from build123d import *

# Parameters (mm, degrees)
SKETCH1_R           = 6.5
BOSS_EXTRUDE1_DEPTH = 22
CAVITY1_START       = 2
CAVITY1_OUTLINE_R   = 5
CAVITY1_OUTLINE_R_2 = 0.75
CAVITY1_DEPTH       = 20
CAVITY1_START_2     = 17
CAVITY1_2_OUTLINE_R = 0.75
CAVITY1_2_DEPTH     = 5
SKETCH2_R           = 0.3
CUT_EXTRUDE1_DEPTH  = 23.011360703


# Read off the part's stored shape, not the designer's step: Cavity1
with BuildPart() as part:
    # Sketch1 → Boss-Extrude1 (new body)
    with BuildSketch(Plane(origin=(0, 0, 0), x_dir=(1, 0, 0), z_dir=(0, 1, 0))):
        with Locations(Location((0, 0, 0), (0, 0, 270))):
            Circle(SKETCH1_R)
    extrude(amount=BOSS_EXTRUDE1_DEPTH)

    # Cavity1 outline → Cavity1 (cut)
    with BuildSketch(Plane(origin=(0, 0, 0), x_dir=(1, 0, 0), z_dir=(0, 1, 0)).offset(CAVITY1_START)):
        Circle(CAVITY1_OUTLINE_R)
        with BuildLine():
            ThreePointArc((-1.5, -2.598076211), (0, -3), (1.5, -2.598076211))
            Line((1.5, -2.598076211), (2, -3.464101615))
            ThreePointArc((2, -3.464101615), (0, -4), (-2, -3.464101615))
            Line((-2, -3.464101615), (-1.5, -2.598076211))
        make_face(mode=Mode.SUBTRACT)
        with BuildLine():
            ThreePointArc((-2.598076211, 1.5), (-3, 0), (-2.598076211, -1.5))
            Line((-2.598076211, -1.5), (-3.464101615, -2))
            ThreePointArc((-3.464101615, -2), (-4, 0), (-3.464101615, 2))
            Line((-3.464101615, 2), (-2.598076211, 1.5))
        make_face(mode=Mode.SUBTRACT)
        Circle(CAVITY1_OUTLINE_R_2, mode=Mode.SUBTRACT)
        with BuildLine():
            ThreePointArc((2.598076211, -1.5), (3, 0), (2.598076211, 1.5))
            Line((2.598076211, 1.5), (3.464101615, 2))
            ThreePointArc((3.464101615, 2), (4, 0), (3.464101615, -2))
            Line((3.464101615, -2), (2.598076211, -1.5))
        make_face(mode=Mode.SUBTRACT)
        with BuildLine():
            ThreePointArc((1.5, 2.598076211), (0, 3), (-1.5, 2.598076211))
            Line((-1.5, 2.598076211), (-2, 3.464101615))
            ThreePointArc((-2, 3.464101615), (0, 4), (2, 3.464101615))
            Line((2, 3.464101615), (1.5, 2.598076211))
        make_face(mode=Mode.SUBTRACT)
    extrude(amount=CAVITY1_DEPTH, mode=Mode.SUBTRACT)

    # Cavity1 2 outline → Cavity1 2 (cut)
    with BuildSketch(Plane(origin=(0, 0, 0), x_dir=(1, 0, 0), z_dir=(0, 1, 0)).offset(CAVITY1_START_2)):
        Circle(CAVITY1_2_OUTLINE_R)
    extrude(amount=CAVITY1_2_DEPTH, mode=Mode.SUBTRACT)

    # Sketch2 → Cut-Extrude1 (cut, through all)
    with BuildSketch(Plane(origin=(0, 2, 0), x_dir=(1, 0, 0), z_dir=(0, 1, 0))):
        with Locations(Location((0, 4.5, 0), (0, 0, 270))):
            Circle(SKETCH2_R)
        with Locations(Location((4.5, 0, 0), (0, 0, 270))):
            Circle(SKETCH2_R)
        with Locations(Location((0, -4.5, 0), (0, 0, 270))):
            Circle(SKETCH2_R)
        with Locations(Location((-4.5, 0, 0), (0, 0, 270))):
            Circle(SKETCH2_R)
    extrude(amount=-CUT_EXTRUDE1_DEPTH, mode=Mode.SUBTRACT)


solid = part.part
The listing builds one solid part. Answer for the finished solid, in the listing's coordinates (mm). A direction names the side the tool comes from. Coordinates: 2 decimals unless noted, no trailing zeros. Loops run counter-clockwise (first coordinate to the right, second up) from the corner with the lowest first, then second, coordinate; pieces in that order, holes last.
1) Determine the mould class of faces 3 (the face through (-3.955, 10.846, -5.158)), 4 (the face through (-3, 12, 0)), 5 (the face through (-3.4, 22, 0)) for opening direction X: pulls with the +X half, pulls with the -X half, needs draft (parallel to the pull), parting line crosses it, or undercut.
2) Find section B-B on z = 0. Write down the section's boundary in (x, y).
3) Find section A-A on y = 14.5. Write down the section's boundary in (x, z).
4) Find the intervals of material crossed by L1, parallel to X at y = 14, z = 0; L2, parallel to X at y = 0.75, z = 0; L3, parallel to Z at x = 1, y = 3, in increasing order.
5) Find section D-D on x = -4.5. Write down the section's boundary in (y, z), then the cut area to 3 significant figures.
6) A tool of negligible diameter and unlimited length cuts with its end or side. For faces 1 (the face through (1.754, 11.86, -3.037)), 2 (the face through (0, 0, 0)), from which of +Z, -Z, +X, -X, +Y, -Y can it reach the whole face along a straight path? Write none if from no direction.
7) Flat-ended cylindrical pins translate along their axes: pin 1 Ø5 at (x, z) = (1, 0) entering from +Y; pin 2 Ø1 at (y, z) = (5.5, -2.5) entering from +X; pin 3 Ø2 at (y, z) = (3.5, 4) entering from +X; pin 4 Ø1.5 at (x, y) = (-5, 16) entering from +Z. Find the tip coordinate at first contact, or state that the pin passes through.
8) Find section C-C on x = 0. Write down the section's boundary in (y, z), then the cut area to 3 significant figures.
Values:
1. face 3: parting line crosses it
1. face 4: undercut
1. face 5: needs draft
2. outline: (-6.5, 0) - (-4.8, 0) - (-4.8, 2) - (-5, 2) - (-5, 22) - (-6.5, 22) - close; (-4.2, 0) - (4.2, 0) - (4.2, 2) - (4, 2) - (4, 22) - (3, 22) - (3, 2) - (0.75, 2) - (0.75, 17) - (-0.75, 17) - (-0.75, 2) - (-3, 2) - (-3, 22) - (-4, 22) - (-4, 2) - (-4.2, 2) - close; (4.8, 0) - (6.5, 0) - (6.5, 22) - (5, 22) - (5, 2) - (4.8, 2) - close
3. outline: circle Ø13 at (0, 0); (-3.46, -2) - (-2.6, -1.5) arc R3 cw to (-2.6, 1.5) - (-3.46, 2) arc R4 ccw to start; (-2, -3.46) arc R4 ccw to (2, -3.46) - (1.5, -2.6) arc R3 cw to (-1.5, -2.6) - close; (-2, 3.46) - (-1.5, 2.6) arc R3 cw to (1.5, 2.6) - (2, 3.46) arc R4 ccw to start; circle Ø1.5 at (0, 0); (2.6, -1.5) - (3.46, -2) arc R4 ccw to (3.46, 2) - (2.6, 1.5) arc R3 cw to start; hole circle Ø10 at (0, 0)
4. L1: x = -6.5 to -5, -4 to -3, -0.75 to 0.75, 3 to 4, 5 to 6.5
4. L2: x = -6.5 to -4.8, -4.2 to 4.2, 4.8 to 6.5
4. L3: z = -6.42 to -4.9, -3.87 to -2.83, 2.83 to 3.87, 4.9 to 6.42
5. outline: (0, -4.69) - (22, -4.69) - (22, -2.18) - (2, -2.18) - (2, -0.3) - (0, -0.3) - close; (0, 0.3) - (2, 0.3) - (2, 2.18) - (22, 2.18) - (22, 4.69) - (0, 4.69) - close
5. area: 118 mm2
6. face 1: +Y
6. face 2: +Z, -Z, +X, -X, -Y
7. pin 1: stops at y = 22
7. pin 2: stops at x = 6.18
7. pin 3: stops at x = 5.77
7. pin 4: stops at z = 4.92
8. outline: (0, -6.5) - (22, -6.5) - (22, -5) - (2, -5) - (2, -4.8) - (0, -4.8) - close; (0, -4.2) - (2, -4.2) - (2, -4) - (22, -4) - (22, -3) - (2, -3) - (2, -0.75) - (17, -0.75) - (17, 0.75) - (2, 0.75) - (2, 3) - (22, 3) - (22, 4) - (2, 4) - (2, 4.2) - (0, 4.2) - close; (0, 4.8) - (2, 4.8) - (2, 5) - (22, 5) - (22, 6.5) - (0, 6.5) - close
8. area: 146 mm2
